```python
from build123d import *

# Parameters (mm, degrees)
CROQUIS1_R              = 1.5
SALIENTE_EXTRUIR1_DEPTH = 3
REDONDEO1_R             = 1


with BuildPart() as part:
    # Croquis1 → Saliente-Extruir1 (new body)
    with BuildSketch(Plane(origin=(0, 0, 0), x_dir=(1, 0, 0), z_dir=(0, 1, 0))):
        Polygon((32.802827881, -15.07231132), (32.802827881, -5.07231132), (15.302827881, -5.07231132), (15.302827881, 14.537092733), (-14.697172119, 14.537092733), (-14.697172119, -5.07231132), (-32.197172119, -5.07231132), (-32.197172119, -15.07231132), align=None)
        with Locations(Location((29.302827881, -10.07231132, 0), (0, 0, 270))):
            Circle(CROQUIS1_R, mode=Mode.SUBTRACT)
        with Locations(Location((-28.697172119, -10.07231132, 0), (0, 0, 90))):
            Circle(CROQUIS1_R, mode=Mode.SUBTRACT)
        with Locations(Location((-10.697172119, 6.389486457, 0), (0, 0, 270))):
            Circle(CROQUIS1_R, mode=Mode.SUBTRACT)
        with Locations(Location((11.302827881, 6.389486457, 0), (0, 0, 90))):
            Circle(CROQUIS1_R, mode=Mode.SUBTRACT)
        with Locations(Location((0.302827881, 0.389486457, 0), (0, 0, 270))):
            Circle(CROQUIS1_R, mode=Mode.SUBTRACT)
    extrude(amount=SALIENTE_EXTRUIR1_DEPTH)

    # Redondeo1
    redondeo1_edges = [part.edges().sort_by_distance(p)[0] for p in [
        (-14.697172119, 1.5, 5.07231132),
        (-14.697172119, 1.5, -14.537092733),
        (15.302827881, 1.5, -14.537092733),
        (15.302827881, 1.5, 5.07231132),
        (32.802827881, 1.5, 5.07231132),
        (32.802827881, 1.5, 15.07231132),
        (-32.197172119, 1.5, 15.07231132),
        (-32.197172119, 1.5, 5.07231132),
    ]]
    fillet(redondeo1_edges, radius=REDONDEO1_R)


solid = part.part
```
Read the model definition and answer for the solid it produces. Units are mm, in the model's axes. A direction names the side the tool comes from. Coordinates: 2 decimals unless noted, no trailing zeros. Write each loop counter-clockwise with the first axis right and the second up, starting at its lowest first coordinate (ties: lowest second). Pieces come first, ordered by that corner, then holes. Notation, with made-up numbers: (50, -37.75) - (108, -37.75) arc R16 cw to (108, -10.75) - close; hole circle Ø5 at (64.5, -27). An arc over 180 degrees is marked (long way). Answer as a JSON object with one key per item and string values. Group by question number.
1. A cutting plane is placed at D-D (z = -9.25). Determine the outline of the cut face in (x, y), plus the area to 3 significant figures.
2. Each of these flat-tipped pins is pushed along its axis until it touches: P1, Ø0.9, axis at x = -22.5, y = 2, coming from the -Z side; P2, Ø1.5, axis at y = 1, z = -6.5, coming from the +X side; P3, Ø2.5, axis at x = -28.7, z = 10.07, coming from the -Y side; P4, Ø1, axis at y = 1, z = -8.5, coming from the -X side. Where does it stop, or does it pass through?
3. A cutting plane is placed at B-B (x = 1). Determine the outline of the cut face in (y, z), plus the area to 3 significant figures.
4. A cutting plane is placed at C-C (y = 2). Determine the outline of the cut face in (x, z).
5. The mould has two halves that part along X. Classify faces 4 (the flat face through (-14.697, 1, -5)), 5 (the flat face through (0, 0, 3)), 6 (the cylindrical face through (-9.432, 1.479, -5.583)): +X half, -X half, draft (parallel to the pull), parting line (faces both ways), or undercut.
6. Consider L1, parallel to Z at x = 29.5, y = 2.8; L2, parallel to X at y = 1.85, z = 10.5; L3, parallel to Z at x = 16.5, y = 2.75. Determine where each line is inside the solid, lowest interval first. Write a range as [from, to].
7. A cutting plane is placed at A-A (z = 10.5). Determine the outline of the cut face in (x, y).
8. Which of the six approach directions +Z, -Z, +X, -X, +Y, -Y give full straight-line access (tool end or side, diameter ignored) to faces 1 (the flat face through (-23, 1, 5.072)), 2 (the flat face through (24, 1, 5.072)), 3 (the flat face through (0, 3, 3))?
Worked out:
{
 "1": {"outline": "(-14.7, 0) - (15.3, 0) - (15.3, 3) - (-14.7, 3) - close", "area": "90.0 mm²"},
 "2": {"P1": "stops at z = 5.07", "P2": "stops at x = 15.3", "P3": "passes through", "P4": "stops at x = -14.7"},
 "3": {"outline": "(0, -14.54) - (3, -14.54) - (3, -1.72) - (0, -1.72) - close; (0, 0.94) - (3, 0.94) - (3, 15.07) - (0, 15.07) - close", "area": "80.9 mm²"},
 "4": {"outline": "(-32.2, 6.07) arc R1 ccw to (-31.2, 5.07) - (-15.7, 5.07) arc R1 cw to (-14.7, 4.07) - (-14.7, -13.54) arc R1 ccw to (-13.7, -14.54) - (14.3, -14.54) arc R1 ccw to (15.3, -13.54) - (15.3, 4.07) arc R1 cw to (16.3, 5.07) - (31.8, 5.07) arc R1 ccw to (32.8, 6.07) - (32.8, 14.07) arc R1 ccw to (31.8, 15.07) - (-31.2, 15.07) arc R1 ccw to (-32.2, 14.07) - close; hole circle Ø3 at (-28.7, 10.07); hole circle Ø3 at (-10.7, -6.39); hole circle Ø3 at (0.3, -0.39); hole circle Ø3 at (11.3, -6.39); hole circle Ø3 at (29.3, 10.07)"},
 "5": {"face 4": "-X half", "face 5": "draft", "face 6": "undercut"},
 "6": {"L1": "z = [5.07, 8.59], [11.56, 15.07]", "L2": "x = [-32.2, -30.13], [-27.26, 27.87], [30.74, 32.8]", "L3": "z = [5.07, 15.07]"},
 "7": {"outline": "(-32.2, 0) - (-30.13, 0) - (-30.13, 3) - (-32.2, 3) - close; (-27.26, 0) - (27.87, 0) - (27.87, 3) - (-27.26, 3) - close; (30.74, 0) - (32.8, 0) - (32.8, 3) - (30.74, 3) - close"},
 "8": {"face 1": "-Z, -X, +Y, -Y", "face 2": "-Z, +X, +Y, -Y", "face 3": "+Z, -Z, +X, -X, +Y"}
}
